Verification items for the finished model (mm, model axes). A direction names the side the tool comes from. Round coordinates to 2 decimals unless told otherwise and drop trailing zeros. Write each loop counter-clockwise with the first axis right and the second up, starting at its lowest first coordinate (ties: lowest second). Pieces come first, ordered by that corner, then holes. Notation, with made-up numbers: (57, 10) - (109, 10) arc R13 ccw to (109, 28) - close; hole circle Ø10 at (57.5, 60). An arc over 180 degrees is marked (long way). Answer as a JSON object with one key per item and string values.
```python
from build123d import *

# Parameters (mm, degrees)
BOSS_EXTRUDE1_DEPTH = 30
FILLET1_R           = 10
FILLET2_R           = 20
FILLET3_R           = 15
FILLET4_R           = 15
SKETCH2_R           = 5
BOSS_EXTRUDE2_DEPTH = 20
SKETCH3_R           = 15
BOSS_EXTRUDE3_DEPTH = 30
FILLET5_R           = 10
SKETCH4_R           = 5
BOSS_EXTRUDE4_DEPTH = 20
SKETCH5_R           = 15
BOSS_EXTRUDE5_DEPTH = 30
FILLET6_R           = 10


with BuildPart() as part:
    # Sketch1 → Boss-Extrude1 (new body)
    with BuildSketch(Plane(origin=(0, 0, 0), x_dir=(0, 0, -1), z_dir=(1, 0, 0))):
        Polygon((-224.956890143, -152.027957955), (-77.928932188, -5), (80, -5), (80, 5), (-82.071067812, 5), (-232.027957955, -144.956890143), align=None)
    extrude(amount=BOSS_EXTRUDE1_DEPTH)

    # Fillet1
    fillet1_edges = [part.edges().sort_by_distance(p)[0] for p in [
        (15, -5, 77.928932188),
    ]]
    fillet(fillet1_edges, radius=FILLET1_R)

    # Fillet2
    fillet2_edges = [part.edges().sort_by_distance(p)[0] for p in [
        (15, 5, 82.071067812),
    ]]
    fillet(fillet2_edges, radius=FILLET2_R)

    # Fillet3
    fillet3_edges = [part.edges().sort_by_distance(p)[0] for p in [
        (30, -148.492424049, 228.492424049),
        (0, -148.492424049, 228.492424049),
    ]]
    fillet(fillet3_edges, radius=FILLET3_R - 0.0001)  # a hair under: the kernel refuses the full size

    # Fillet4
    fillet4_edges = [part.edges().sort_by_distance(p)[0] for p in [
        (30, 0, -80),
        (0, 0, -80),
    ]]
    fillet(fillet4_edges, radius=FILLET4_R - 0.0001)  # a hair under: the kernel refuses the full size

    # Sketch2 → Boss-Extrude2 (add)
    with BuildSketch(Plane(origin=(0, 43.535533906, 43.535533906), x_dir=(1, 0, 0), z_dir=(0, 0.7071067811865471, 0.7071067811865479))):
        with Locations(Location((15, -251.568542495, 0), (0, 0, 270))):
            Circle(SKETCH2_R)
    extrude(amount=BOSS_EXTRUDE2_DEPTH)

    # Sketch3 → Boss-Extrude3 (add)
    with BuildSketch(Plane(origin=(0, 57.67766953, 57.67766953), x_dir=(1, 0, 0), z_dir=(0, 0.7071067811865471, 0.7071067811865479))):
        with Locations(Location((15, -251.568542495, 0), (0, 0, 270))):
            Circle(SKETCH3_R)
    extrude(amount=BOSS_EXTRUDE3_DEPTH)

    # Fillet5
    fillet5_edges = [part.edges().sort_by_distance(p)[0] for p in [
        (15, -88.388347648, 246.170093579),
    ]]
    fillet(fillet5_edges, radius=FILLET5_R)

    # Sketch4 → Boss-Extrude4 (add)
    with BuildSketch(Plane.XZ.offset(5)):
        with Locations(Location((15, -65, 0), (0, 0, 90))):
            Circle(SKETCH4_R)
    extrude(amount=BOSS_EXTRUDE4_DEPTH)

    # Sketch5 → Boss-Extrude5 (add)
    with BuildSketch(Plane(origin=(0, 5, 0), x_dir=(1, 0, 0), z_dir=(0, 1, 0))):
        with Locations(Location((15, 65, 0), (0, 0, 270))):
            Circle(SKETCH5_R)
    extrude(amount=BOSS_EXTRUDE5_DEPTH)

    # Fillet6
    fillet6_edges = [part.edges().sort_by_distance(p)[0] for p in [
        (15, 35, -80),
    ]]
    fillet(fillet6_edges, radius=FILLET6_R)


solid = part.part
```
1. Material ranges on probe 1 along Y at (x, z) = (6.5, 69.5); probe 2 along Z at (x, y) = (2.5, -104); probe 3 along Z at (x, y) = (23, -98.5), recorded low to high. Write a range as from..to.
Completed:
{"probe 1": "y = -5..5", "probe 2": "z = 176.93..191.07, 240.05..256.3", "probe 3": "z = 171.43..185.57, 239.33..255.59"}
2. Mould release check, pull along Y, two halves, no side actions. Record for faces 4 (the face through (10.564, -129.01, 230.025)), 5 (the face through (0.357, 14.86, -68.252)), 6 (the face through (9.255, -123.034, 252.333)): released by +Y, released by -Y, zero draft, split by the parting line, or undercut.
Completed:
{"face 4": "undercut", "face 5": "zero draft", "face 6": "split by the parting line"}
3. Cross-section at A-A (z = 171.5). Record the boundary of the cut face in (x, y).
Completed:
{"outline": "(0, -98.57) - (30, -98.57) - (30, -84.43) - (0, -84.43) - close"}
4. Go/stop test with flat-tipped pins: pin 1 (1 mm diameter, centred on x = 22.5, y = -66.5, fed in from +Z); pin 2 (3 mm diameter, centred on x = 13, y = 10, fed in from -Z); pin 3 (12 mm diameter, centred on x = 23.5, z = 69.5, fed in from -Y). Record where each tip stops, or that it passes through.
Completed:
{"pin 1": "stops at z = 154.07", "pin 2": "stops at z = -79.99", "pin 3": "stops at y = -5.15"}
5. Access from +Z, -Z, +X, -X, +Y, -Y to the whole of each face (thin tool, end or side, straight path). Record for faces 1 (the face through (8.543, -120.06, 235.415)), 2 (the face through (15.21, -5.78, 77.66)), 3 (the face through (15, -25, -65)).
Completed:
{"face 1": "none", "face 2": "+X, -X, -Y", "face 3": "-Z, +X, -X, -Y"}
